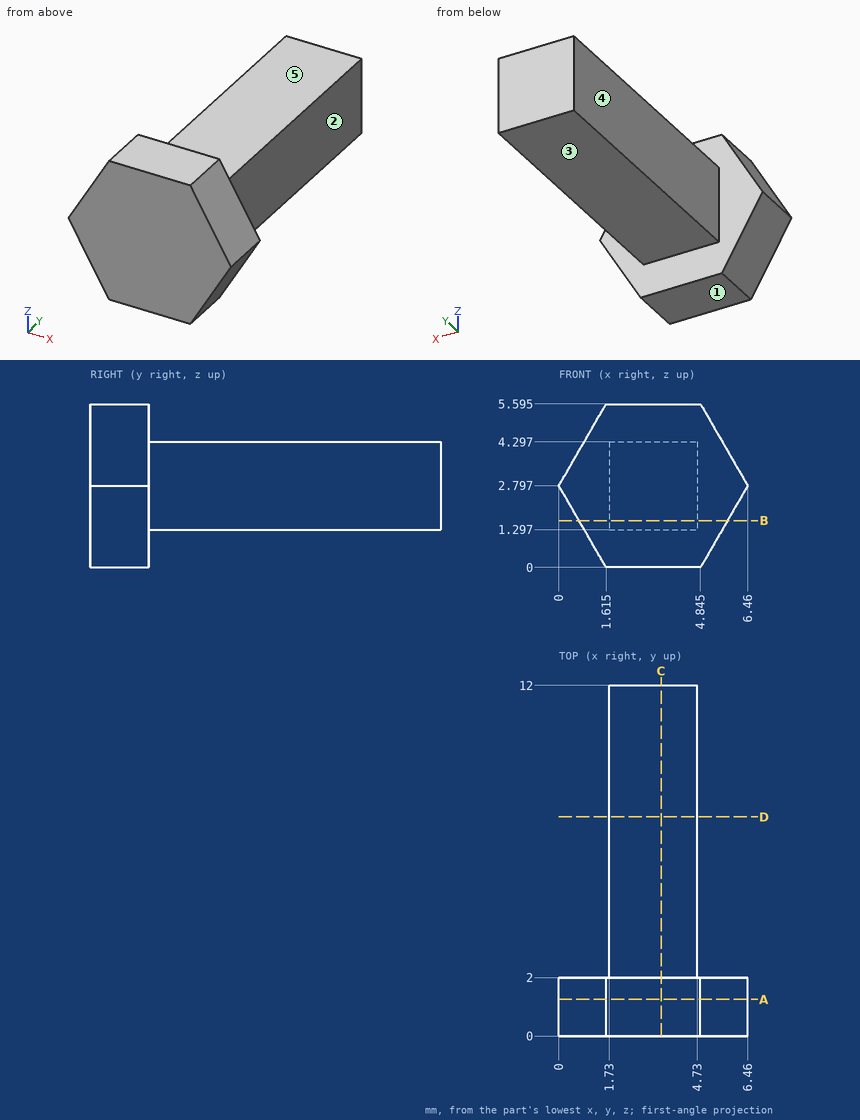
The figure shows three views and two pictorial views of one solid part (mm, origin at its lowest corner). Answer the questions. A direction names the side the tool comes from. Give positions to 0.01 mm unless a question says otherwise; leave off trailing zeros. Order: outer loops, then holes, each group sorted by start corner. A loop starts at its lowest first (then second) coordinate and runs counter-clockwise, first axis right, second up. Notation, with made-up numbers: (72.25, -15.5) -> (111.25, -15.5) arc R9 ccw to (111.25, 0.5) -> close; hole circle Ø4 at (9, -9). An arc over 180 degrees is marked (long way). Answer as a JSON object with one key per item and string values. Group by question number.
Item 1: A tool of negligible diameter and unlimited length cuts with its end or side. For the marked faces 1, 2, 3, 4 and 5, from which of +Z, -Z, +X, -X, +Y, -Y can it reach the whole face along a straight path? Write none if from no direction.
Item 2: The part is cut by section B-B on z = 1.6. Write down the section's boundary in (x, y).
Item 3: The part is cut by section A-A on y = 1.25. Write down the section's boundary in (x, z) (1 decimal), and give its area (3 significant figures).
Item 4: The part is cut by section D-D on y = 7.5. Write down the section's boundary in (x, z).
Item 5: Flat-ended cylindrical pins translate along their axes: pin 1 (1.5 mm diameter, centred on x = 3, y = 7, fed in from +Z); pin 2 (1.5 mm diameter, centred on x = 2.5, y = 8.5, fed in from -Z); pin 3 (2 mm diameter, centred on y = 7.5, z = 5, fed in from +X). Find the tip coordinate at first contact, or state that the pin passes through.
Item 6: Consider L1, parallel to Z at x = 3.5, y = 8.5; L2, parallel to X at y = 11, z = 3.95; L3, parallel to Y at x = 4, z = 0.7. Determine where each line is inside the solid, lowest interval first. Write a range as from..to.
Item 7: The part is cut by section C-C on x = 3.5. Write down the section's boundary in (y, z) (1 decimal).
Result set:
{
 "1": {"face 1": "-Z, +X, -X, +Y, -Y", "face 2": "+Z, -Z, +X, +Y", "face 3": "-Z, +X, -X, +Y", "face 4": "+Z, -Z, -X, +Y", "face 5": "+Z, +X, -X, +Y"},
 "2": {"outline": "(0.69, 0) -> (5.77, 0) -> (5.77, 2) -> (4.73, 2) -> (4.73, 12) -> (1.73, 12) -> (1.73, 2) -> (0.69, 2) -> close"},
 "3": {"outline": "(0, 2.8) -> (1.6, 0) -> (4.8, 0) -> (6.5, 2.8) -> (4.8, 5.6) -> (1.6, 5.6) -> close", "area": "27.1 mm²"},
 "4": {"outline": "(1.73, 1.3) -> (4.73, 1.3) -> (4.73, 4.3) -> (1.73, 4.3) -> close"},
 "5": {"pin 1": "z = 4.3", "pin 2": "z = 1.3", "pin 3": "x = 4.73"},
 "6": {"L1": "1.3..4.3", "L2": "1.73..4.73", "L3": "0..2"},
 "7": {"outline": "(0, 0) -> (2, 0) -> (2, 1.3) -> (12, 1.3) -> (12, 4.3) -> (2, 4.3) -> (2, 5.6) -> (0, 5.6) -> close"}
}
